from build123d import *

# Parameters (mm, degrees)
SKETCH_R        = 50
SKETCH_R_2      = 8
SKETCH_R_3      = 6
PAD_DEPTH       = 10
POCKET_DEPTH    = 2
CYLINDER_R      = 3.5
CYLINDER_DEPTH  = 12
SKETCH002_R     = 1.5
POCKET001_DEPTH = 10
BOX_W           = 15
BOX_H           = 1.6
BOX_DEPTH       = 4


with BuildPart() as part:
    # Sketch → Pad (new body)
    with BuildSketch(Plane.XY):
        Circle(SKETCH_R)
        with Locations((0, 35)):
            Circle(SKETCH_R_2, mode=Mode.SUBTRACT)
        with Locations((24.748737, 24.748737)):
            Circle(SKETCH_R_2, mode=Mode.SUBTRACT)
        with Locations((35, 0)):
            Circle(SKETCH_R_2, mode=Mode.SUBTRACT)
        with Locations((24.748737, -24.748737)):
            Circle(SKETCH_R_2, mode=Mode.SUBTRACT)
        with Locations((0, -35)):
            Circle(SKETCH_R_2, mode=Mode.SUBTRACT)
        with Locations((-24.748737, -24.748737)):
            Circle(SKETCH_R_2, mode=Mode.SUBTRACT)
        with Locations((-35, 0)):
            Circle(SKETCH_R_2, mode=Mode.SUBTRACT)
        with Locations((-24.748737, 24.748737)):
            Circle(SKETCH_R_2, mode=Mode.SUBTRACT)
        with Locations((-7.653669, -18.477591)):
            Circle(SKETCH_R_3, mode=Mode.SUBTRACT)
        with Locations((7.653669, -18.477591)):
            Circle(SKETCH_R_3, mode=Mode.SUBTRACT)
        with Locations((18.477591, -7.653669)):
            Circle(SKETCH_R_3, mode=Mode.SUBTRACT)
        with Locations((18.477591, 7.653669)):
            Circle(SKETCH_R_3, mode=Mode.SUBTRACT)
        with Locations((7.653669, 18.477591)):
            Circle(SKETCH_R_3, mode=Mode.SUBTRACT)
        with Locations((-7.653669, 18.477591)):
            Circle(SKETCH_R_3, mode=Mode.SUBTRACT)
        with Locations((-18.477591, 7.653669)):
            Circle(SKETCH_R_3, mode=Mode.SUBTRACT)
        with Locations((-18.477591, -7.653669)):
            Circle(SKETCH_R_3, mode=Mode.SUBTRACT)
    extrude(amount=PAD_DEPTH)

    # Sketch001 (on Face19 of Pad) → Pocket (cut)
    with BuildSketch(Plane.XY.offset(10)):
        Polygon((43.884278, 18.177463), (18.177463, 43.884278), (-18.177463, 43.884278), (-43.884278, 18.177463), (-43.884278, -18.177463), (-18.177463, -43.884278), (18.177463, -43.884278), (43.884278, -18.177463), align=None)
    extrude(amount=-POCKET_DEPTH, mode=Mode.SUBTRACT)

    # Cone → Cone (revolve)
    with BuildSketch(Plane(origin=(0, 0, 8), x_dir=(1, 0, 0), z_dir=(0, -1, 0))):
        Polygon((0, 0), (10, 0), (5, 8), (0, 8), align=None)
    revolve(axis=Axis((0, 0, 8), (0, 0, 1)))

    # Cylinder → Cylinder (cut)
    with BuildSketch(Plane(origin=(0, 0, 16), x_dir=(-1, 0, 0), z_dir=(0, 0, -1))):
        Circle(CYLINDER_R)
    extrude(amount=CYLINDER_DEPTH, mode=Mode.SUBTRACT)

    # Sketch002 (on Face32 of Cylinder) → Pocket001 (cut)
    with BuildSketch(Plane(origin=(0, 0, 4), x_dir=(-1, 0, 0), z_dir=(0, 0, 1))):
        Circle(SKETCH002_R)
    extrude(amount=-POCKET001_DEPTH, mode=Mode.SUBTRACT)

    # Box → Box (cut)
    with BuildSketch(Plane(origin=(-7, -0.75, 15), x_dir=(1, 0, 0), z_dir=(0, 0, 1))):
        with Locations((7.5, 0.8)):
            Rectangle(BOX_W, BOX_H)
    extrude(amount=BOX_DEPTH, mode=Mode.SUBTRACT)


solid = part.part
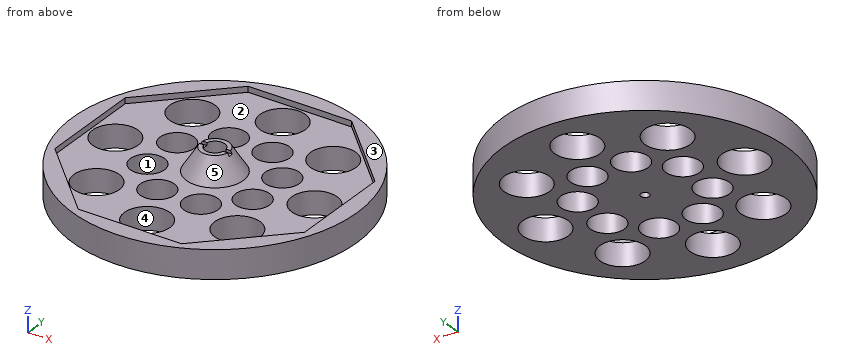
Can you work these out from the model? Positions are in its coordinate system, mm. Face numbers are marked on the shaded views. A direction names the side the tool comes from. Coordinates: 2 decimals unless noted, no trailing zeros. Write each loop counter-clockwise with the first axis right and the second up, starting at its lowest first coordinate (ties: lowest second). Pieces come first, ordered by that corner, then holes. Notation, with made-up numbers: (35.25, 4.25) -> (54.25, 4.25) arc R12 cw to (54.25, 13.25) -> close; hole circle Ø6 at (17, -26). An arc over 180 degrees is marked (long way). Write each question's results on one line, items separated by ' | '. Start each with the question number.
Item 1: Please list where these lines run through material, in increasing order: probe 1 along Y at (x, z) = (14.5, 1); probe 2 along X at (y, z) = (-1, 8.25); probe 3 along Y at (x, z) = (-32, 7).
Item 2: If we section it at D-D, the plane z = 2.25: Count the separate pieces of the cut face and the enclosed holes in it, and give its area (3 significant figures).
Item 3: If we section it at A-A, the plane x = 0: Write out the boundary of the cut face in (y, z).
Item 4: If we section it at B-B, the plane y = -35: Write out the boundary of the cut face in (x, z), and give its area (3 significant figures).
Item 5: I'm going to push flat-ended pins straight in: P1, Ø18.5, axis at x = -35, y = 0, coming from the +Z side; P2, Ø1.5, axis at x = -2, y = 7, coming from the +Z side; P3, Ø10, axis at x = -33.5, y = 11, coming from the +Z side. Where does each tip first touch, or does it pass through?
Item 6: On a 3-axis mill with a long thin cutter (end or side, diameter ignored), from which of +Z, -Z, +X, -X, +Y, -Y can I reach the whole of each face in a straight line? I mean the marked faces 1 and 2. Say none if no direction works.
Item 7: Thinking about a two-plate mould opening in X: for the marked faces 3, 4 and 5, which applies, released by +X, released by -X, zero draft, split by the parting line, or undercut?
Answer block:
1) probe 1: -47.85 to -12.15, -3.16 to 3.16, 12.15 to 47.85 | probe 2: -49.99 to -43.88, -9.79 to -3.35, 3.35 to 9.79, 43.88 to 49.99 | probe 3: -38.42 to -28.13, -21.37 to -7.42, 7.42 to 21.37, 28.13 to 38.42
2) separate pieces: 1 | enclosed holes: 17 | area: 5,330 mm²
3) outline: (-50, 0) -> (-43, 0) -> (-43, 8) -> (-43.88, 8) -> (-43.88, 10) -> (-50, 10) -> close; (-27, 0) -> (-1.5, 0) -> (-1.5, 4) -> (-3.5, 4) -> (-3.5, 16) -> (-5, 16) -> (-10, 8) -> (-27, 8) -> close; (1.5, 0) -> (27, 0) -> (27, 8) -> (10, 8) -> (5, 16) -> (3.5, 16) -> (3.5, 4) -> (1.5, 4) -> close; (43, 0) -> (50, 0) -> (50, 10) -> (43.88, 10) -> (43.88, 8) -> (43, 8) -> close
4) outline: (-35.71, 0) -> (-8, 0) -> (-8, 8) -> (-27.06, 8) -> (-27.06, 10) -> (-35.71, 10) -> close; (8, 0) -> (35.71, 0) -> (35.71, 10) -> (27.06, 10) -> (27.06, 8) -> (8, 8) -> close | area: 478 mm²
5) P1: z = 10 | P2: z = 13.55 | P3: z = 8
6) face 1: +Z, -Z | face 2: +Z
7) face 3: zero draft | face 4: undercut | face 5: undercut
